Build history of the part. All positions in model axes, mm. Face numbers are marked on the shaded views. A direction names the side the tool comes from. Give positions to 0.01 mm unless a question says otherwise; leave off trailing zeros. Loops run counter-clockwise (first coordinate to the right, second up) from the corner with the lowest first, then second, coordinate; pieces in that order, holes last. Notation, with made-up numbers: M 2.25,-31 L 9.25,-31 A27 ccw 9.25,-10 Z; hole C -9.75,-6 d11. An arc over 180 degrees is marked long. Put each result on its own line as item: value.
Autodesk Inventor part; units mm, degrees
ref_plane "YZ Plane" through (0, 0, 0) normal (1, 0, 0) x (0, 1, 0)
ref_plane "XZ Plane" through (0, 0, 0) normal (0, 1, 0) x (-1, 0, 0)
sketch "Sketch2" plane through (0, 0, 0) normal (1, 0, 0) x (0, 1, 0)
  line L0 (23, 25) -> (0, 25)
  line L1 (0, 25) -> (0, -25)
  line L2 (0, -25) -> (23, -25)
  line L3 (23, -25) -> (23, 25)
  line L4 (20, 22) -> (3, 22)
  line L5 (3, 22) -> (3, -22)
  line L6 (3, -22) -> (20, -22)
  line L7 (20, -22) -> (20, 22)
  line L8 (0, -35) -> (0, 35)
  line L9 (-4.6, 0) -> (27.6, 0)
  point P0 (0, 0)
  dimension "d8" = 50
  dimension "d9" = 23
  dimension "d10" = 3
  dimension "d11" = 3
  dimension "d12" = 3
  dimension "d13" = 17
extrude "Extrusion3" add sketch "Sketch2" along normal blind 3
extrude "Extrusion4" add sketch "Sketch2" along normal blind 53 contours L3 L9 L7 L4 L5 L1 L0 | L3 L2 L1 L9 L5 L6 L7
sketch "Sketch5" plane through (53, 0, 0) normal (1, 0, 0) x (0, 0, -1)
  line L0 (25, 0) -> (25, 23)
  line L1 (25, 23) -> (-25, 23)
  line L2 (-25, 23) -> (-25, 0)
  line L3 (-25, 0) -> (25, 0)
  line L4 (22, 3) -> (-22, 3)
  line L5 (-22, 3) -> (-22, 20)
  line L6 (-22, 20) -> (22, 20)
  line L7 (22, 20) -> (22, 3)
  line L8 (22, 11.5) -> (30, 11.5)
  line L9 (25, 0) -> (25, 23)
  circle A0 centre (30, 11.5) radius 4.75
  line L10 (30, 6.75) -> (25, 6.75)
  line L11 (30, 16.25) -> (25, 16.25)
  circle A1 centre (30, 11.5) radius 2.1
  point P0 (0, 0)
  point P1 (25, 6.75)
  dimension "d32" = 9.5
  dimension "d33" = 5
  dimension "d39" = 4.2
extrude "Extrusion7" add sketch "Sketch5" against normal blind 8 contours L0 L8 A0 L10 | L0 L11 A0 L8 | A0
sketch "Sketch6" plane through (45, 0, 0) normal (-1, 0, 0) x (0, 0, 1)
  line L0 (-30, 6.75) -> (-25, 6.75)
  line L1 (-25, 16.25) -> (-25, 6.75)
  line L2 (-25, 16.25) -> (-30, 16.25)
  arc A0 (-30, 16.25) -> (-30, 6.75) centre (-30, 11.5) ccw
  line L3 (-25.8431, 11.5) -> (-27.9215, 7.9)
  line L4 (-27.9215, 7.9) -> (-32.0785, 7.9)
  line L5 (-32.0785, 7.9) -> (-34.1569, 11.5)
  line L6 (-34.1569, 11.5) -> (-32.0785, 15.1)
  line L7 (-32.0785, 15.1) -> (-27.9215, 15.1)
  line L8 (-27.9215, 15.1) -> (-25.8431, 11.5)
  point P0 (0, 0)
  dimension "d36" = 7.2
extrude "Extrusion8" cut sketch "Sketch6" against normal blind 4 contours L3 L4 L5 L6 L7 L8
mirror "Mirror1" about plane through (0, 0, 0) normal (0, 0, 1) of "Extrusion7", "Extrusion8"
equation "\"d12\" = d11"
properties part number "pudelko_baza"
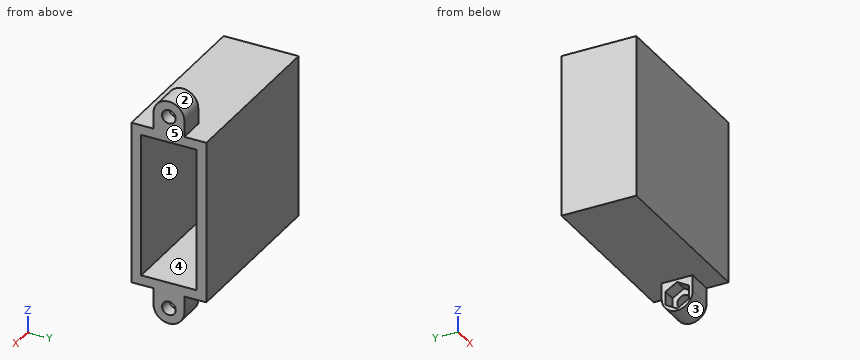
Q1. Slice it at C-C (y = 10.25). List the corners of the cut face in (x, z).
Here are the results:
outline: M 0,-25 L 45,-25 L 45,-26.56 L 49,-26.56 L 49,-28.31 L 53,-28.31 L 53,-22 L 3,-22 L 3,22 L 53,22 L 53,28.31 L 49,28.31 L 49,26.56 L 45,26.56 L 45,25 L 0,25 Z; M 45,-34.58 L 53,-34.58 L 53,-31.69 L 49,-31.69 L 49,-33.44 L 45,-33.44 Z; M 45,33.44 L 49,33.44 L 49,31.69 L 53,31.69 L 53,34.58 L 45,34.58 Z
Q2. Slice it at A-A (x = 21.5). List the corners of the cut face in (y, z).
Here are the results:
outline: M 0,-25 L 23,-25 L 23,25 L 0,25 Z; hole M 3,-22 L 20,-22 L 20,22 L 3,22 Z
Q3. Slice it at D-D (y = 1.75). List the corners of the cut face in (x, z), and give its area (3 significant figures).
Here are the results:
outline: M 0,-25 L 53,-25 L 53,25 L 0,25 Z
area: 2,650 mm²
Q4. Tool access for the marked faces 4 and 5: list every direction of +Z, -Z, +X, -X, +Y, -Y with a clear straight run to the whole face (end or side of a thin tool).
Here are the results:
face 4: +X
face 5: +Z, -Z, +X, +Y, -Y
Q5. Drop flat-ended pins along their axis: pin 1 Ø5 at (x, y) = (33, 16) entering from +Z; pin 2 Ø6 at (y, z) = (10.5, 29.5) entering from -X; pin 3 Ø13.5 at (x, y) = (27.5, 15) entering from -Z; pin 4 Ø4 at (y, z) = (11.5, 30) entering from -X. Give the stop position or say it passes through.
Here are the results:
pin 1: z = 25
pin 2: x = 45
pin 3: z = -25
pin 4: through
Q6. Slice it at B-B (z = 9.5). List the corners of the cut face in (x, y), and give its area (3 significant figures).
Here are the results:
outline: M 0,0 L 53,0 L 53,3 L 3,3 L 3,20 L 53,20 L 53,23 L 0,23 Z
area: 369 mm²
Q7. Probe line 1 (Z direction, x = 26.5, y = 14.5); line 2 (Y direction, x = 8, z = -20); line 3 (X direction, y = 6, z = -12). List the from-to ranges inside material, lowest first. Write a range as from..to.
Here are the results:
line 1: -25..-22, 22..25
line 2: 0..3, 20..23
line 3: 0..3
Q8. Mould opens along Z. For the marked faces 1, 2 and 3 say: pulls with the +Z half, pulls with the -Z half, needs draft (parallel to the pull), parting line crosses it, or undercut.
Here are the results:
face 1: undercut
face 2: pulls with the +Z half
face 3: pulls with the -Z half
